Read the model definition and answer for the solid it produces. Units are mm, in the model's axes. A direction names the side the tool comes from. Coordinates: 2 decimals unless noted, no trailing zeros. Order: outer loops, then holes, each group sorted by start corner. A loop starts at its lowest first (then second) coordinate and runs counter-clockwise, first axis right, second up. Notation, with made-up numbers: M 33.25,77.25 L 44.25,77.25 A26 ccw 44.25,100.25 Z; hole C -27.5,47 d1. An arc over 180 degrees is marked long. Use a Markdown table: item, result. Add a question column.
1) Find the intervals of material crossed by probe 1 along Z at (x, y) = (0, 3) (3 decimals); probe 2 along Z at (x, y) = (-3.5, 1.5) (3 decimals); probe 3 along Y at (x, z) = (-5.75, 4), in increasing order. Write a range as [from, to].
2) Each of these flat-tipped pins is pushed along its axis until it touches: pin 1 Ø2 at (x, y) = (-4.5, 2.5) entering from +Z (3 decimals); pin 2 Ø5 at (y, z) = (7, 4) entering from -X; pin 3 Ø3.5 at (x, y) = (-1, 5.5) entering from -Z (3 decimals). Where does it stop, or does it pass through?
3) Find section D-D on x = -2.75. Write down the section's boundary in (y, z) (3 decimals).
4) Find section A-A on x = 0. Write down the section's boundary in (y, z) (3 decimals), plus the area to 3 significant figures.
5) Find section C-C on z = -1.25. Write down the section's boundary in (x, y), plus the area to 3 significant figures.
6) For faces 4 (the face through (3, 7.5, -6)), 5 (the face through (0, 4, 6.285)), 6 (the face through (5.418, 3.698, 3.186)), 7 (the face through (5.468, 3.698, -3.099)), determine the directions among +Z, -Z, +X, -X, +Y, -Y from which every point of the face is accessible in a straight line to the end or side of a thin tool.
7) The mould has two halves that part along X. Classify faces 1 (the face through (-6.05, -0.64, -4.64)), 2 (the face through (-5.418, 3.698, -3.186)), 3 (the face through (0, 4.3, -1.6)): released by +X, released by -X, zero draft, split by the parting line, or undercut.
8) Find section B-B on y = 0.75. Write down the section's boundary in (x, z) (3 decimals), plus the area to 3 significant figures.
from build123d import *

# Parameters (mm, degrees)
BOSS_EXTRUDE1_DEPTH = 7.5
SKETCH2_R           = 6.1
BOSS_EXTRUDE2_DEPTH = 2.3
SKETCH3_R           = 7.625
BOSS_EXTRUDE3_DEPTH = 1.3
CUT_EXTRUDE1_DEPTH  = 12.1


with BuildPart() as part:
    # Sketch1 → Boss-Extrude1 (new body)
    with BuildSketch(Plane(origin=(0, 0, 0), x_dir=(1, 0, 0), z_dir=(0, 1, 0))):
        Polygon((7.257292884, 0), (3.628646442, 6.285), (-3.628646442, 6.285), (-7.257292884, 0), (-3.628646442, -6.285), (3.628646442, -6.285), align=None)
    extrude(amount=BOSS_EXTRUDE1_DEPTH)

    # Sketch2 → Boss-Extrude2 (add)
    with BuildSketch(Plane(origin=(0, 7.5, 0), x_dir=(1, 0, 0), z_dir=(0, 1, 0))):
        Circle(SKETCH2_R)
    extrude(amount=BOSS_EXTRUDE2_DEPTH)

    # Sketch3 → Boss-Extrude3 (add)
    with BuildSketch(Plane.XZ):
        Circle(SKETCH3_R)
    extrude(amount=BOSS_EXTRUDE3_DEPTH)

    # Sketch4 → Cut-Extrude1 (cut, through all)
    with BuildSketch(Plane(origin=(0, 9.8, 0), x_dir=(1, 0, 0), z_dir=(0, 1, 0))):
        with BuildLine():
            Line((-1.3, -0.932737905), (1.3, -0.932737905))
            ThreePointArc((1.3, -0.932737905), (0, 1.6), (-1.3, -0.932737905))
        make_face()
    extrude(amount=-CUT_EXTRUDE1_DEPTH, mode=Mode.SUBTRACT)


solid = part.part
Check result:
| question | item | result |
|---|---|---|
| 1 | probe 1 | z = [-6.285, -1.6], [0.933, 6.285] |
| 1 | probe 2 | z = [-6.285, 6.285] |
| 1 | probe 3 | y = [-1.3, 0] |
| 2 | pin 1 | stops at z = 6.285 |
| 2 | pin 2 | stops at x = -6.39 |
| 2 | pin 3 | stops at z = -6.285 |
| 3 | outline | M -1.3,-7.112 L 0,-7.112 L 0,-6.285 L 7.5,-6.285 L 7.5,-5.445 L 9.8,-5.445 L 9.8,5.445 L 7.5,5.445 L 7.5,6.285 L 0,6.285 L 0,7.112 L -1.3,7.112 Z |
| 4 | outline | M -1.3,-7.625 L 0,-7.625 L 0,-6.285 L 7.5,-6.285 L 7.5,-6.1 L 9.8,-6.1 L 9.8,-1.6 L -1.3,-1.6 Z; M -1.3,0.933 L 9.8,0.933 L 9.8,6.1 L 7.5,6.1 L 7.5,6.285 L 0,6.285 L 0,7.625 L -1.3,7.625 Z |
| 4 | area | 114 mm2 |
| 5 | outline | M -7.52,-1.3 L -1,-1.3 L -1,9.8 L -5.97,9.8 L -5.97,7.5 L -6.54,7.5 L -6.54,0 L -7.52,0 Z; M 1,-1.3 L 7.52,-1.3 L 7.52,0 L 6.54,0 L 6.54,7.5 L 5.97,7.5 L 5.97,9.8 L 1,9.8 Z |
| 5 | area | 123 mm2 |
| 6 | face 4 | +Y |
| 6 | face 5 | +Z, +X, -X, +Y |
| 6 | face 6 | +Z, +X, +Y |
| 6 | face 7 | -Z, +X, +Y |
| 7 | face 1 | split by the parting line |
| 7 | face 2 | released by -X |
| 7 | face 3 | undercut |
| 8 | outline | M -7.257,0 L -3.629,-6.285 L 3.629,-6.285 L 7.257,0 L 3.629,6.285 L -3.629,6.285 Z; hole M -1.3,0.933 A1.6 ccw long 1.3,0.933 Z |
| 8 | area | 130 mm2 |
